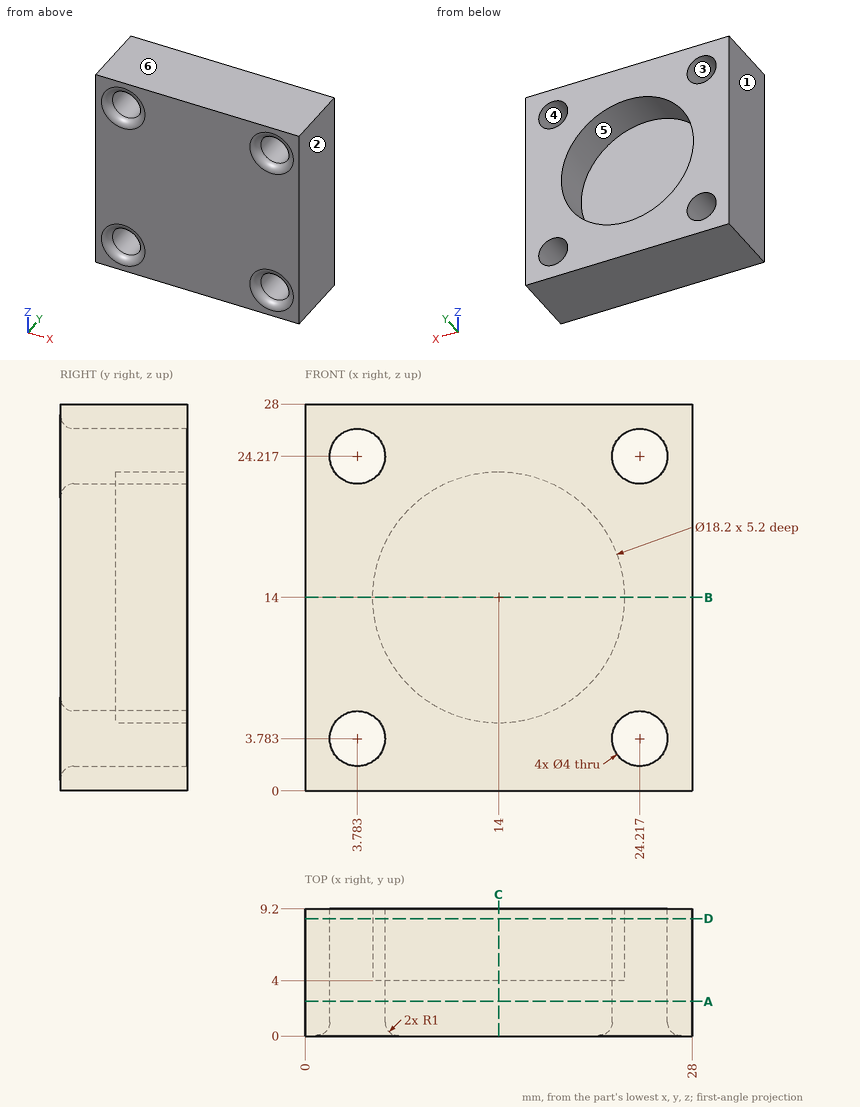
Could you check a few things on this drawing? It's one solid part, dimensions in mm from its lowest x, y, z. A direction names the side the tool comes from. Round coordinates to 2 decimals unless told otherwise and drop trailing zeros. Write each loop counter-clockwise with the first axis right and the second up, starting at its lowest first coordinate (ties: lowest second). Pieces come first, ordered by that corner, then holes.
Q1. If we section it at D-D on y = 8.5: Write out the boundary of the cut face in (x, z).
Q2. Please list where these lines run through material, in increasing order: probe 1 along X at (y, z) = (8.5, 24.25); probe 2 along Z at (x, y) = (25, 6.25); probe 3 along X at (y, z) = (6.2, 14).
Q3. If we section it at C-C on x = 14: Write out the boundary of the cut face in (y, z), plus the area to 3 significant figures.
Q4. If we mould it in two halves opening along X, with no side actions, what happens to the marked faces 1, 2, 3 and 4? For each: +X half, -X half, draft (parallel to the pull), parting line (faces both ways), or undercut.
Q5. Will these pins go through, and if not, where does the flat tip stop? P1, Ø2, axis at y = 5.5, z = 3, coming from the -X side; P2, Ø9, axis at x = 11.5, z = 15.5, coming from the +Y side; P3, Ø5, axis at x = 24.22, z = 3.78, coming from the -Y side.
Q6. Which directions (+Z, -Z, +X, -X, +Y, -Y) give clear straight access to the entire face, cutting with the end or side of a thin tool? Please do the marked faces 5 and 6.
Q7. If we section it at A-A on y = 2.5: Write out the boundary of the cut face in (x, z), plus the area to 3 significant figures.
Q8. If we section it at B-B on z = 14: Write out the boundary of the cut face in (x, y).
Answer below:
1. outline: (0, 0) - (28, 0) - (28, 28) - (0, 28) - close; hole circle Ø4 at (3.78, 3.78); hole circle Ø4 at (3.78, 24.22); hole circle Ø18.2 at (14, 14); hole circle Ø4 at (24.22, 3.78); hole circle Ø4 at (24.22, 24.22)
2. probe 1: x = 0 to 1.78, 5.78 to 22.22, 26.22 to 28
2. probe 2: z = 0 to 1.94, 5.62 to 22.38, 26.06 to 28
2. probe 3: x = 0 to 4.9, 23.1 to 28
3. outline: (0, 0) - (9.2, 0) - (9.2, 4.9) - (4, 4.9) - (4, 23.1) - (9.2, 23.1) - (9.2, 28) - (0, 28) - close
3. area: 163 mm2
4. face 1: -X half
4. face 2: +X half
4. face 3: undercut
4. face 4: undercut
5. P1: stops at x = 0
5. P2: stops at y = 4
5. P3: stops at y = 0.13
6. face 5: +Y
6. face 6: +Z, +X, -X, +Y, -Y
7. outline: (0, 0) - (28, 0) - (28, 28) - (0, 28) - close; hole circle Ø4 at (3.78, 3.78); hole circle Ø4 at (3.78, 24.22); hole circle Ø4 at (24.22, 3.78); hole circle Ø4 at (24.22, 24.22)
7. area: 734 mm2
8. outline: (0, 0) - (28, 0) - (28, 9.2) - (23.1, 9.2) - (23.1, 4) - (4.9, 4) - (4.9, 9.2) - (0, 9.2) - close
